Geometry: final body of the model. Coordinates: model frame, mm. A direction names the side the tool comes from. Give positions to 0.01 mm unless a question says otherwise; leave off trailing zeros. Order: outer loops, then holes, each group sorted by start corner. A loop starts at its lowest first (then second) coordinate and runs counter-clockwise, first axis right, second up. Notation, with made-up numbers: (66, 7) - (71, 7) arc R35 cw to (71, 44) - close; hole circle Ø10 at (-26.75, -1.75). An arc over 180 degrees is marked (long way). Use one line per item in the form item = value.
from build123d import *

# Parameters (mm, degrees)
SKETCH1_W                                     = 40
SKETCH1_H                                     = 8
CUT_EXTRUDE1_DEPTH                            = 58.131427428
SKETCH3_W                                     = 13
SKETCH3_H                                     = 2
BOSS_EXTRUDE1_DEPTH                           = 3.5
CUT_EXTRUDE2_DEPTH                            = 6
CUT_EXTRUDE3_DEPTH                            = 6
CUT_EXTRUDE4_DEPTH                            = 6
CUT_EXTRUDE5_DEPTH                            = 6
F_7_0_7_DIAMETER_HOLE1_D                      = 7
F_2_5_2_5_DIAMETER_HOLE1_D                    = 2.5
F_2_5_2_5_DIAMETER_HOLE1_DEPTH                = 11.5
F_8_8_8_8_DIAMETER_HOLE1_D                    = 8.8
F_8_8_8_8_DIAMETER_HOLE1_DEPTH                = 11.5
CBORE_FOR_M4_HEX_HEAD_MACHINE_SCREW1_AT_COUNT = 2
CBORE_FOR_M4_HEX_HEAD_MACHINE_SCREW1_AT_PITCH = 36.57489953
CBORE_FOR_M4_HEX_HEAD_MACHINE_SCREW1_2_COUNT  = 2
CBORE_FOR_M4_HEX_HEAD_MACHINE_SCREW1_2_PITCH  = 62.370456693
CBORE_FOR_M4_HEX_HEAD_MACHINE_SCREW1_3_COUNT  = 2
CBORE_FOR_M4_HEX_HEAD_MACHINE_SCREW1_3_PITCH  = 31.779334982
CBORE_FOR_M4_HEX_HEAD_MACHINE_SCREW1_4_COUNT  = 2
CBORE_FOR_M4_HEX_HEAD_MACHINE_SCREW1_4_PITCH  = 59.684811505
CBORE_FOR_M4_HEX_HEAD_MACHINE_SCREW1_5_COUNT  = 2
CBORE_FOR_M4_HEX_HEAD_MACHINE_SCREW1_5_PITCH  = 70
F_5_0_5_DIAMETER_HOLE1_D                      = 5
FILLET1_R                                     = 0.5


with BuildPart() as part:
    # Sketch1 → Revolve1 (revolve)
    with BuildSketch(Plane.XY, mode=Mode.PRIVATE) as revolve1_sk:
        with Locations((20, 4)):
            Rectangle(SKETCH1_W, SKETCH1_H)
    revolve(revolve1_sk.sketch.rotate(Axis((0, 8, 0), (0, -1, 0)), 270), axis=Axis((0, 8, 0), (0, -1, 0)))

    # Sketch2 → Cut-Extrude1 (cut, through all)
    with BuildSketch(Plane(origin=(0, 8, 0), x_dir=(-1, 0, 0), z_dir=(0, 1, 0))):
        Polygon((-6.069687354, -20.679550025), (-10.040517244, -10.851401166), (-15.163753313, -12.921322899), (-11.192923423, -22.749471758), align=None)
    extrude(amount=-CUT_EXTRUDE1_DEPTH, mode=Mode.SUBTRACT)

    # Sketch3 → Boss-Extrude1 (add)
    with BuildSketch(Plane.XZ):
        Rectangle(SKETCH3_W, SKETCH3_H)
    extrude(amount=BOSS_EXTRUDE1_DEPTH)

    # Sketch4 → Cut-Extrude2 (cut)
    with BuildSketch(Plane.XZ):
        Polygon((-2.29496732, 26.975), (-4.58993464, 23), (-2.29496732, 19.025), (2.29496732, 19.025), (4.58993464, 23), (2.29496732, 26.975), align=None)
    extrude(amount=-CUT_EXTRUDE2_DEPTH, mode=Mode.SUBTRACT)

    # Sketch5 → Cut-Extrude3 (cut)
    with BuildSketch(Plane.XZ):
        Polygon((-26.975, -2.29496732), (-23, -4.58993464), (-19.025, -2.29496732), (-19.025, 2.29496732), (-23, 4.58993464), (-26.975, 2.29496732), align=None)
    extrude(amount=-CUT_EXTRUDE3_DEPTH, mode=Mode.SUBTRACT)

    # Sketch6 → Cut-Extrude4 (cut)
    with BuildSketch(Plane.XZ):
        Polygon((2.29496732, -26.975), (4.58993464, -23), (2.29496732, -19.025), (-2.29496732, -19.025), (-4.58993464, -23), (-2.29496732, -26.975), align=None)
    extrude(amount=-CUT_EXTRUDE4_DEPTH, mode=Mode.SUBTRACT)

    # Sketch7 → Cut-Extrude5 (cut)
    with BuildSketch(Plane.XZ):
        Polygon((26.975, 2.29496732), (23, 4.58993464), (19.025, 2.29496732), (19.025, -2.29496732), (23, -4.58993464), (26.975, -2.29496732), align=None)
    extrude(amount=-CUT_EXTRUDE5_DEPTH, mode=Mode.SUBTRACT)

    # Ø7.0 (7) Diameter Hole1 (through all)
    with Locations(Plane(origin=(0, 0, 0), x_dir=(-1, 0, 0), z_dir=(0, -1, 0))):
        with Locations((4.3, -12.88), (4.3, 12.88), (-4.3, 12.88), (-4.3, -12.88)):
            Hole(F_7_0_7_DIAMETER_HOLE1_D / 2)

    # Ø2.5 (2.5) Diameter Hole1
    with Locations(Plane(origin=(0, 8, 0), x_dir=(1, 0, 0), z_dir=(0, 1, 0))):
        with Locations((25, -7.5), (25, 7.5), (-25, 7.5), (-25, -7.5)):
            Hole(F_2_5_2_5_DIAMETER_HOLE1_D / 2, depth=F_2_5_2_5_DIAMETER_HOLE1_DEPTH)

    # Ø8.8 (8.8) Diameter Hole1
    with Locations(Plane(origin=(0, 8, 0), x_dir=(1, 0, 0), z_dir=(0, 1, 0))):
        with Locations((33, 0), (-33, 0)):
            Hole(F_8_8_8_8_DIAMETER_HOLE1_D / 2, depth=F_8_8_8_8_DIAMETER_HOLE1_DEPTH)

    # Sketch14 → CBORE for M4 Hex Head Machine Screw1 (revolve, cut)
    with BuildSketch(Plane(origin=(-31.185228347, 8, 15.889667491), x_dir=(0, 0, 1), z_dir=(1, 0, 0))):
        Polygon((0, 0), (0, 11.5), (2.4, 11.5), (2.4, 5), (4, 5), (4, 1.32), (5.32, 0), align=None)
    cbore_for_m4_hex_head_machine_screw1 = revolve(axis=Axis((-31.185228347, 14.35, 15.889667491), (0, -1, 0)), mode=Mode.SUBTRACT)

    # CBORE for M4 Hex Head Machine Screw1 at: CBORE for M4 Hex Head Machine Screw1 ×2
    with Locations(*[Vector(0.8526401643540931, 0, 0.5224985647159477) * (i * CBORE_FOR_M4_HEX_HEAD_MACHINE_SCREW1_AT_PITCH) for i in range(1, CBORE_FOR_M4_HEX_HEAD_MACHINE_SCREW1_AT_COUNT)]):
        add(cbore_for_m4_hex_head_machine_screw1, mode=Mode.SUBTRACT)

    # CBORE for M4 Hex Head Machine Screw1 2: CBORE for M4 Hex Head Machine Screw1 ×2
    with Locations(*[(i * CBORE_FOR_M4_HEX_HEAD_MACHINE_SCREW1_2_PITCH, 0, 0) for i in range(1, CBORE_FOR_M4_HEX_HEAD_MACHINE_SCREW1_2_COUNT)]):
        add(cbore_for_m4_hex_head_machine_screw1, mode=Mode.SUBTRACT)

    # CBORE for M4 Hex Head Machine Screw1 3: CBORE for M4 Hex Head Machine Screw1 ×2
    with Locations(*[(0, 0, -i * CBORE_FOR_M4_HEX_HEAD_MACHINE_SCREW1_3_PITCH) for i in range(1, CBORE_FOR_M4_HEX_HEAD_MACHINE_SCREW1_3_COUNT)]):
        add(cbore_for_m4_hex_head_machine_screw1, mode=Mode.SUBTRACT)

    # CBORE for M4 Hex Head Machine Screw1 4: CBORE for M4 Hex Head Machine Screw1 ×2
    with Locations(*[Vector(0.5224985647159471, 0, -0.8526401643540933) * (i * CBORE_FOR_M4_HEX_HEAD_MACHINE_SCREW1_4_PITCH) for i in range(1, CBORE_FOR_M4_HEX_HEAD_MACHINE_SCREW1_4_COUNT)]):
        add(cbore_for_m4_hex_head_machine_screw1, mode=Mode.SUBTRACT)

    # CBORE for M4 Hex Head Machine Screw1 5: CBORE for M4 Hex Head Machine Screw1 ×2
    with Locations(*[Vector(0.8910065241883662, 0, -0.45399049973955025) * (i * CBORE_FOR_M4_HEX_HEAD_MACHINE_SCREW1_5_PITCH) for i in range(1, CBORE_FOR_M4_HEX_HEAD_MACHINE_SCREW1_5_COUNT)]):
        add(cbore_for_m4_hex_head_machine_screw1, mode=Mode.SUBTRACT)

    # Ø5.0 (5) Diameter Hole1 (through all)
    with Locations(Plane(origin=(0, 6, 0), x_dir=(-1, 0, 0), z_dir=(0, -1, 0))):
        with Locations((-23, 0), (0, 23), (23, 0), (0, -23)):
            Hole(F_5_0_5_DIAMETER_HOLE1_D / 2)

    # Fillet1
    fillet1_edges = [part.edges().sort_by_distance(p)[0] for p in [
        (0, 0, 40),
    ]]
    fillet(fillet1_edges, radius=FILLET1_R)


solid = part.part
(1) Contact query for flat-ended pins moving along their axis: pin 1 Ø2 at (x, z) = (8, 29.5) entering from -Y; pin 2 Ø9 at (x, z) = (2, -36.5) entering from +Y; pin 3 Ø3 at (x, y) = (-21.5, 5.5) entering from +Z; pin 4 Ø4 at (x, y) = (18.5, 3.5) entering from +Z. Output: stop coordinate, or through.
Computed values:
pin_1 = 0
pin_2 = 8
pin_3 = 34.64
pin_4 = 36.44
(2) Reachability of faces 1 (the face through (8.67, 4.06, -21.73)), 2 (the face through (0, 5, 31)), 3 (the face through (-3.46, 2.96, 21.04)) from +Z, -Z, +X, -X, +Y, -Y: full face, straight path, thin tool, end or side. Return the list, or none.
Computed values:
face_1 = +Y, -Y
face_2 = +Y
face_3 = -Y
(3) Pull-direction query (Z, two-part tool) for faces 4 (the face through (35.09, 4.87, 15.02)), 5 (the face through (1, 8, -1)); classes: released by +Z, released by -Z, zero draft, split by the parting line, or undercut.
Computed values:
face_4 = undercut
face_5 = zero draft
(4) Cut plane A-A on y = -1.75. Output: boundary loops of the cut face in (x, z), plus the area to 3 significant figures.
Computed values:
outline = (-6.5, -1) - (6.5, -1) - (6.5, 1) - (-6.5, 1) - close
area = 26.0 mm²
(5) Cut plane B-B on z = -7.5. Give the number of separate pieces and of enclosed holes in the cut face, plus the area to 3 significant figures.
Computed values:
separate_pieces = 3
enclosed_holes = 0
area = 589 mm²
(6) Ray query, line 1 along Z through (x, y) = (0, 1.95) (3 decimals); line 2 along Z through (x, y) = (6, 6); line 3 along Z through (x, y) = (-25, 5.5). Return the intervals inside material, ascending.
Computed values:
line_1 = -40 to -37.4, -32.6 to -26.975, -19.025 to 19.025, 26.975 to 32.6, 37.4 to 40
line_2 = -39.55 to -15.94, -9.82 to 9.82, 15.94 to 39.55
line_3 = -31.22 to -8.75, -6.25 to -3.44, 3.44 to 6.25, 8.75 to 31.22
